```python
from build123d import *

# Parameters (mm, degrees)
F1_DEPTH = 152.4
F2_W     = 16.4605937898
F2_H     = 16.4605937898
F3_DEPTH = 12.7
F5_DEPTH = 25.4


with BuildPart() as f1:
    # F0 (on Front) → F1 (new body)
    with BuildSketch(Plane.XZ):
        Polygon((15.4824422158, -26.1103501737), (30.3534476601, 0.3530131847), (14.8710054442, 26.4633633584), (-15.4824422158, 26.1103501737), (-30.3534476601, -0.3530131847), (-14.8710054442, -26.4633633584), align=None)
    extrude(amount=F1_DEPTH)

    # F2 (on face) → F3 (join)
    with BuildSketch(Plane(origin=(0.3057183858, 0, -26.2868567661), x_dir=(0.9999323774, 0, 0.0116292988), z_dir=(0.0116292988, 0, -0.9999323774))):
        with Locations((0, 138.0381435156)):
            Rectangle(F2_W, F2_H)
    extrude(amount=F3_DEPTH)

    # F4 (on face) → F5 (cut)
    with BuildSketch(Plane.XZ.offset(146.2684404105)):
        Polygon((-3.4819418117, -39.031766442), (-7.8319489835, -34.2993618355), (-7.7763298602, -39.0817105412), align=None)
    extrude(amount=-F5_DEPTH, mode=Mode.SUBTRACT)


solid = f1.part
```
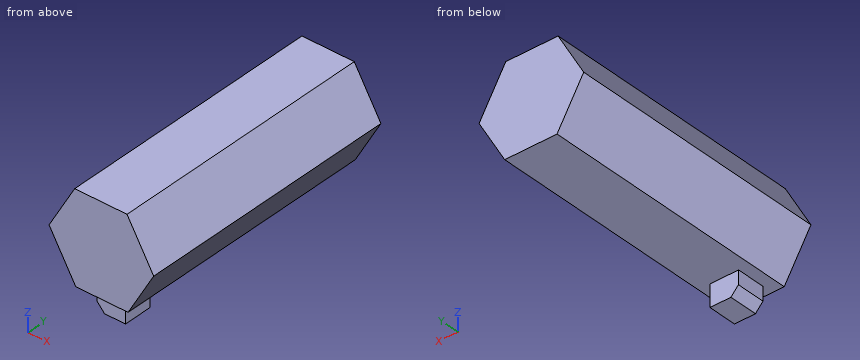
CAD build for the part. Positions are in the model's coordinates, mm. Coordinates: 2 decimals unless noted, no trailing zeros. Write each loop counter-clockwise with the first axis right and the second up, starting at its lowest first coordinate (ties: lowest second). Pieces come first, ordered by that corner, then holes.
(1) Flat gauge pins, fed straight in: pin 1 (12 mm diameter, centred on y = -40, z = 9, fed in from -X); pin 2 (4 mm diameter, centred on y = -134, z = 15, fed in from -X); pin 3 (5 mm diameter, centred on x = -12, y = -51.5, fed in from -Z). Where does each tip first touch, or does it go through?
(2) Drill centre lines: probe 1 along X at (y, z) = (-133.5, -2); probe 2 along X at (y, z) = (-40.5, 16.5); probe 3 along Z at (x, y) = (19.5, -103). Where is each one in solid material? Low to high.
(3) Cut at B-B, the plane x = -1. List the corners of the cut face in (y, z).
(4) Cut at D-D, the plane x = -23.5. List the corners of the cut face in (y, z), and give its area (3 significant figures).
(5) Cut at A-A, the plane y = -57.5. List the corners of the cut face in (x, z), and give its area (3 significant figures).
(6) Cut at C-C, the plane z = -10.5. List the corners of the cut face in (x, y), and give its area (3 significant figures).
Geometry says:
1. pin 1: stops at x = -28.47
1. pin 2: stops at x = -22.85
1. pin 3: stops at z = -26.46
2. probe 1: x = -29.38 to 29.03
2. probe 2: x = -20.88 to 20.78
2. probe 3: z = -18.96 to 18.66
3. outline: (-152.4, -26.3) - (-146.27, -26.3) - (-146.27, -39) - (-129.81, -39) - (-129.81, -26.3) - (0, -26.3) - (0, 26.28) - (-152.4, 26.28) - close
4. outline: (-152.4, -11.91) - (0, -11.91) - (0, 11.84) - (-152.4, 11.84) - close
4. area: 3,620 mm2
5. outline: (-30.35, -0.35) - (-14.87, -26.46) - (15.48, -26.11) - (30.35, 0.35) - (14.87, 26.46) - (-15.48, 26.11) - close
5. area: 2,390 mm2
6. outline: (-24.34, -152.4) - (24.25, -152.4) - (24.25, 0) - (-24.34, 0) - close
6. area: 7,410 mm2
